```python
from build123d import *

# Parameters (mm, degrees)
F0_R     = 140.5
F1_DEPTH = 20
F0_R_2   = 195
F0_R_3   = 13.5
F2_DEPTH = 10
F4_DEPTH = 25


with BuildPart() as f1:
    # F0 (on Front) → F1 (new body)
    with BuildSketch(Plane.XZ):
        Circle(F0_R)
    extrude(amount=F1_DEPTH)

    # F0 (on Front) → F2 (join)
    with BuildSketch(Plane.XZ):
        Circle(F0_R_2)
        with Locations((-98.45403, -135.510347)):
            Circle(F0_R_3, mode=Mode.SUBTRACT)
        with Locations((-159.301966, -51.760347)):
            Circle(F0_R_3, mode=Mode.SUBTRACT)
        with Locations((0, -167.5)):
            Circle(F0_R_3, mode=Mode.SUBTRACT)
        with Locations((98.45403, -135.510347)):
            Circle(F0_R_3, mode=Mode.SUBTRACT)
        with Locations((159.301966, -51.760347)):
            Circle(F0_R_3, mode=Mode.SUBTRACT)
        with Locations((-159.301966, 51.760347)):
            Circle(F0_R_3, mode=Mode.SUBTRACT)
        with Locations((-98.45403, 135.510347)):
            Circle(F0_R_3, mode=Mode.SUBTRACT)
        Circle(F0_R, mode=Mode.SUBTRACT)
        with Locations((159.301966, 51.760347)):
            Circle(F0_R_3, mode=Mode.SUBTRACT)
        with Locations((0, 167.5)):
            Circle(F0_R_3, mode=Mode.SUBTRACT)
        with Locations((98.45403, 135.510347)):
            Circle(F0_R_3, mode=Mode.SUBTRACT)
    extrude(amount=F2_DEPTH)

    # F3 (on face) → F4 (cut)
    with BuildSketch(Plane.XZ.offset(20)):
        with BuildLine():
            ThreePointArc((81.240384, 15), (89.284381, 19.059115), (90.798076, 27.941176))
            ThreePointArc((90.798076, 27.941176), (0, 95), (-90.798076, 27.941176))
            ThreePointArc((-90.798076, 27.941176), (-89.284381, 19.059115), (-81.240384, 15))
            Line((-81.240384, 15), (81.240384, 15))
        make_face()
        with BuildLine():
            Line((81.240384, -15), (-81.240384, -15))
            ThreePointArc((-81.240384, -15), (-89.284381, -19.059115), (-90.798076, -27.941176))
            ThreePointArc((-90.798076, -27.941176), (0, -95), (90.798076, -27.941176))
            ThreePointArc((90.798076, -27.941176), (89.284381, -19.059115), (81.240384, -15))
        make_face()
    extrude(amount=-F4_DEPTH, mode=Mode.SUBTRACT)


solid = f1.part
```
Verification items for the finished model (mm, model axes). A direction names the side the tool comes from. Coordinates: 2 decimals unless noted, no trailing zeros. Write each loop counter-clockwise with the first axis right and the second up, starting at its lowest first coordinate (ties: lowest second). Pieces come first, ordered by that corner, then holes. Notation, with made-up numbers: M 37,10 L 72,10 A7 ccw 72,17 Z; hole C -22,19.5 d6. An arc over 180 degrees is marked long. Answer as a JSON object with one key per item and string values. Group by question number.
(1) Cross-section at C-C, the plane z = -167.5. Record the cut outline in (x, y), and give its area (3 significant figures).
(2) Cross-section at B-B, the plane x = 0. Record the cut outline in (y, z).
(3) Tool access check on faces 5 (the face through (-111.5, -14.93, -85.49)), 6 (the face through (-2, -20, 2)), 7 (the face through (89.206, -10.14, 18.954)). Record the directions out of +Z, -Z, +X, -X, +Y, -Y that give a thin tool (end or side, any length) a straight path to the whole face; none if there is none.
(4) Cross-section at A-A, the plane z = 0. Record the cut outline in (x, y), and give its area (3 significant figures).
(5) Material ranges on line 1 (Z direction, x = 0, y = -7.5); line 2 (Z direction, x = -65, y = -1); line 3 (Z direction, x = 78, y = -16.25), recorded low to high.
(6) Gauge pin test, flat ends, axial feed: pin 1 (2 mm diameter, centred on x = 86.5, y = -13.5, fed in from +Z); pin 2 (2 mm diameter, centred on x = 154.5, y = -9.5, fed in from +Z); pin 3 (1 mm diameter, centred on y = -7.5, z = -110, fed in from -X). Record the tip position at first contact, or that the pin passes through.
(7) Release check for a two-part mould opening along Z. For faces 1 (the face through (-154.75, -4.93, -118.65)), 2 (the face through (1, -10, -15)), 3 (the face through (-108.404, -4.93, -126.386)), 4 (the face through (-3, 0, 3)) record: +Z half, -Z half, draft (parallel to the pull), parting line (faces both ways), or undercut.
(8) Cross-section at D-D, the plane y = -14.5. Record the cut outline in (x, z), and give its area (3 significant figures).
Reply:
{
 "1": {"outline": "M -99.84,-10 L -13.5,-10 L -13.5,0 L -99.84,0 Z; M 13.5,-10 L 99.84,-10 L 99.84,0 L 13.5,0 Z", "area": "1,730 mm²"},
 "2": {"outline": "M -20,-140.5 L -10,-140.5 L -10,-154 L 0,-154 L 0,-95 L -20,-95 Z; M -20,-15 L 0,-15 L 0,15 L -20,15 Z; M -20,95 L 0,95 L 0,154 L -10,154 L -10,140.5 L -20,140.5 Z; M -10,-195 L 0,-195 L 0,-181 L -10,-181 Z; M -10,181 L 0,181 L 0,195 L -10,195 Z"},
 "3": {"face 5": "-Y", "face 6": "+Z, -Z, +X, -X, -Y", "face 7": "+Y, -Y"},
 "4": {"outline": "M -195,-10 L -140.5,-10 L -140.5,-20 L 140.5,-20 L 140.5,-10 L 195,-10 L 195,0 L -195,0 Z", "area": "6,710 mm²"},
 "5": {"line 1": "-195 to -181, -154 to -95, -15 to 15, 95 to 154, 181 to 195", "line 2": "-183.85 to -69.28, -15 to 15, 69.28 to 183.85", "line 3": "-116.86 to -54.23, -15 to 15, 54.23 to 116.86"},
 "6": {"pin 1": "z = 111.49", "pin 2": "z = 120.26", "pin 3": "x = -161.35"},
 "7": {"face 1": "parting line", "face 2": "undercut", "face 3": "undercut", "face 4": "draft"},
 "8": {"outline": "C 0,0 d281; hole M -90.8,-27.94 A95 ccw 90.8,-27.94 A10 ccw 81.24,-15 L -81.24,-15 A10 ccw Z; hole M -90.8,27.94 A10 ccw -81.24,15 L 81.24,15 A10 ccw 90.8,27.94 A95 ccw Z", "area": "39,500 mm²"}
}
